For this review, use the dimensioned drawing (mm, ordinates from the lowest corner) and the shaded views. A direction names the side the tool comes from. Round coordinates to 2 decimals unless told otherwise and drop trailing zeros. Order: outer loops, then holes, each group sorted by start corner. A loop starts at its lowest first (then second) coordinate and runs counter-clockwise, first axis right, second up. Notation, with made-up numbers: M 22,79 L 46,79 A33 cw 46,109 Z; hole C 48,50 d3. An arc over 180 degrees is marked long. Use a Markdown table: item, result. Add a question column.
1. Consider section C-C on x = 38. State the section outline as (y, z) points (1 decimal), then the cut area to 3 significant figures.
2. Insertion check: P1, Ø1, axis at x = 21, y = 42.5, coming from the -Z side; P2, Ø1.5, axis at y = 35, z = 17, coming from the -X side; P3, Ø12, axis at y = 53, z = 17.5, coming from the -X side; P4, Ø6, axis at y = 46.5, z = 6.5, coming from the -X side. Each pin has a flat end and moves straight along its axis. Give the tip position at first contact, or say it passes through.
3. Consider section B-B on z = 5.5. State the section outline as (x, y) points.
4. For the marked faces 1 and 2, list the 3-axis set-ups (+Z, -Z, +X, -X, +Y, -Y) from which the entire face can be reached by the end or side of a thin tool; tool diameter is ignored.
5. Consider section D-D on x = 70. State the section outline as (y, z) points (1 decimal).
6. To check wall thickness, follow probe 1 along Y at (x, z) = (37.5, 10.75) (1 decimal); probe 2 along Y at (x, z) = (49, 7) (1 decimal); probe 3 along X at (y, z) = (31, 8.25) (1 decimal). State the ranges of each line that lie inside material, in increasing order.
7. Consider section A-A on y = 40. State the section outline as (x, z) points.
8. The part is to be moulded in two halves that separate along X. For the marked faces 3, 4, 5 and 6, say which applies: +X half, -X half, draft (parallel to the pull), parting line (faces both ways), or undercut.
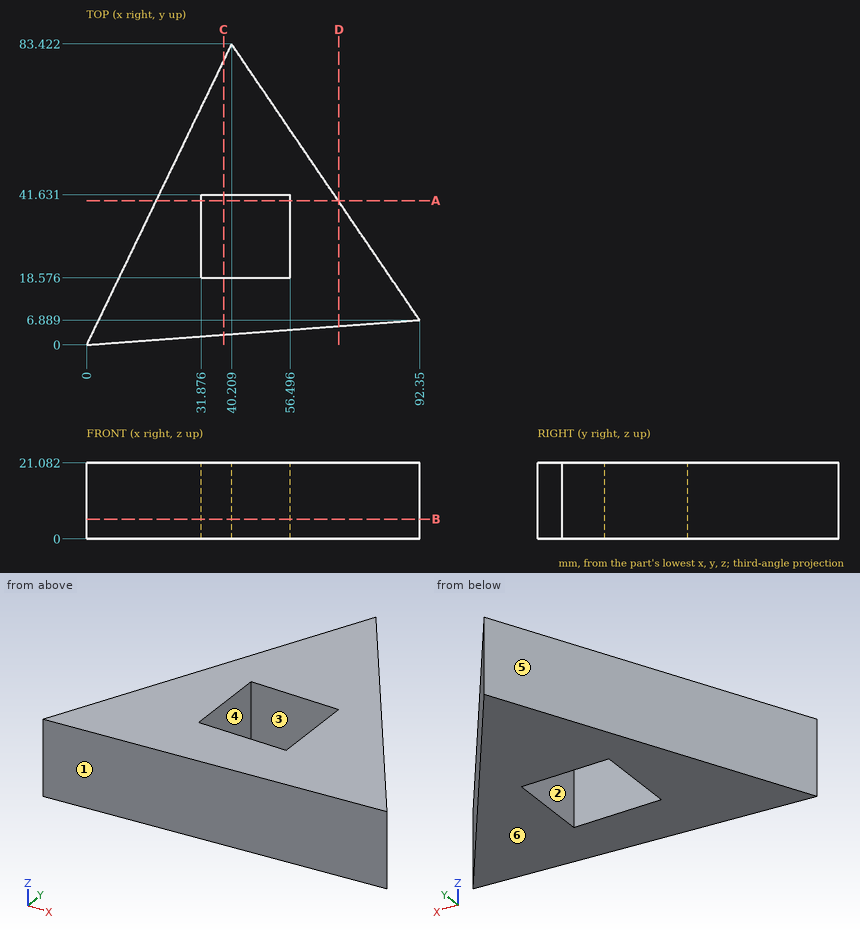
Answer block:
| question | item | result |
|---|---|---|
| 1 | outline | M 2.8,0 L 18.6,0 L 18.6,21.1 L 2.8,21.1 Z; M 41.6,0 L 78.8,0 L 78.8,21.1 L 41.6,21.1 Z |
| 1 | area | 1,120 mm^2 |
| 2 | P1 | z = 0 |
| 2 | P2 | x = 16.51 |
| 2 | P3 | x = 22.65 |
| 2 | P4 | x = 20.97 |
| 3 | outline | M 0,0 L 92.35,6.89 L 40.21,83.42 Z; hole M 31.88,18.58 L 56.5,18.58 L 56.5,41.63 L 31.88,41.63 Z |
| 4 | face 1 | +Z, -Z, +X, -Y |
| 4 | face 2 | +Z, -Z |
| 5 | outline | M 5.2,0 L 39.7,0 L 39.7,21.1 L 5.2,21.1 Z |
| 6 | probe 1 | 2.8 to 18.6, 41.6 to 77.8 |
| 6 | probe 2 | 3.7 to 18.6, 41.6 to 70.5 |
| 6 | probe 3 | 14.9 to 31.9, 56.5 to 75.9 |
| 7 | outline | M 19.28,0 L 31.88,0 L 31.88,21.08 L 19.28,21.08 Z; M 56.5,0 L 69.79,0 L 69.79,21.08 L 56.5,21.08 Z |
| 8 | face 3 | undercut |
| 8 | face 4 | undercut |
| 8 | face 5 | -X half |
| 8 | face 6 | draft |
